Geometry: see drawing. Coordinates: mm, zero at the bounding-box minimum. A direction names the side the tool comes from. Coordinates: 2 decimals unless noted, no trailing zeros. Write each loop counter-clockwise with the first axis right and the second up, starting at its lowest first coordinate (ties: lowest second). Pieces come first, ordered by that corner, then holes. Notation, with made-up numbers: (-32.75, -21.5) - (-17.75, -21.5) arc R11 cw to (-17.75, -13.5) - close; hole circle Ø4 at (-17, -2.5). An arc over 180 degrees is marked (long way). Use a Markdown table: item, result. Add a question column.
Q1. Pin query (flat end, axial travel): P1, Ø3, axis at x = 11.5, z = 19, coming from the +Y side; P2, Ø0.6, axis at x = 12, z = 23, coming from the -Y side; P3, Ø5, axis at y = 21.5, z = 2.5, coming from the -X side. Return the tip coordinate at first contact, or that it passes through.
Q2. Material intervals for probe 1 along Y at (x, z) = (11.5, 3); probe 2 along X at (y, z) = (22, 3.5); probe 3 along X at (y, z) = (32, 12), sorted ascending. Write a range as from..to.
Q3. Section query B-B (z = 13). Return the cut outline in (x, y).
Q4. Section query C-C (x = 2.5). Return the cut outline in (y, z), then the cut area to 3 significant figures.
Q5. Mould query, pull axis Z, two halves, no side actions, for the marked faces 1, 2 and 3. Classes: released by +Z, released by -Z, zero draft, split by the parting line, or undercut.
Q6. Section query A-A (y = 20.3). Return the cut outline in (x, z).
Q7. Set-up query: the marked faces 4, 5, 6, 7 and 8. Return all of +Z, -Z, +X, -X, +Y, -Y with unobstructed straight access to the full face (end or side cutting, diameter ignored); none if empty.
Q8. Section query D-D (y = 9). Return the cut outline in (x, z).
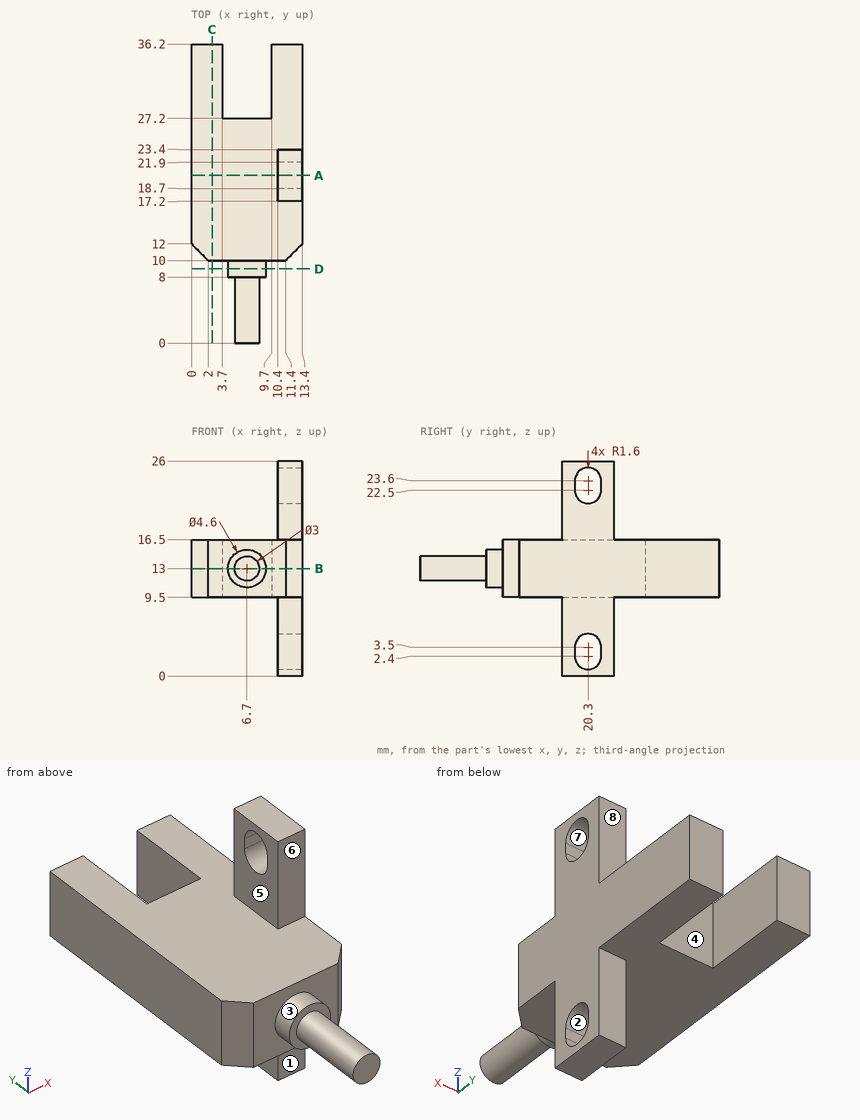
Values follow:
| question | item | result |
|---|---|---|
| 1 | P1 | y = 23.4 |
| 1 | P2 | y = 17.2 |
| 1 | P3 | x = 10.4 |
| 2 | probe 1 | 17.2..18.7, 21.9..23.4 |
| 2 | probe 2 | 10.4..13.4 |
| 2 | probe 3 | 0..3.7, 9.7..13.4 |
| 3 | outline | (0, 12) - (2, 10) - (4.4, 10) - (4.4, 8) - (5.2, 8) - (5.2, 0) - (8.2, 0) - (8.2, 8) - (9, 8) - (9, 10) - (11.4, 10) - (13.4, 12) - (13.4, 36.2) - (9.7, 36.2) - (9.7, 27.2) - (3.7, 27.2) - (3.7, 36.2) - (0, 36.2) - close |
| 4 | outline | (10, 9.5) - (36.2, 9.5) - (36.2, 16.5) - (10, 16.5) - close |
| 4 | area | 183 mm2 |
| 5 | face 1 | zero draft |
| 5 | face 2 | undercut |
| 5 | face 3 | split by the parting line |
| 6 | outline | (0, 9.5) - (10.4, 9.5) - (10.4, 5.1) - (13.4, 5.1) - (13.4, 20.9) - (10.4, 20.9) - (10.4, 16.5) - (0, 16.5) - close; (10.4, 0) - (13.4, 0) - (13.4, 0.8) - (10.4, 0.8) - close; (10.4, 25.2) - (13.4, 25.2) - (13.4, 26) - (10.4, 26) - close |
| 7 | face 4 | +Z, -Z, +Y |
| 7 | face 5 | +Z, -X, +Y, -Y |
| 7 | face 6 | +Z, +X, -X, -Y |
| 7 | face 7 | +X, -X |
| 7 | face 8 | +Z, +X, -X, +Y |
| 8 | outline | circle Ø4.6 at (6.7, 13) |
